Read the model definition and answer for the solid it produces. Units are mm, in the model's axes. Face numbers are marked on the shaded views. A direction names the side the tool comes from. Coordinates: 2 decimals unless noted, no trailing zeros. Order: outer loops, then holes, each group sorted by start corner. A loop starts at its lowest first (then second) coordinate and runs counter-clockwise, first axis right, second up. Notation, with made-up numbers: (-29.75, -7.75) - (-10.75, -7.75) arc R21 cw to (-10.75, 16.25) - close; hole circle Ø3 at (50.5, 19.5). An arc over 180 degrees is marked (long way). Write item = value, one per line.
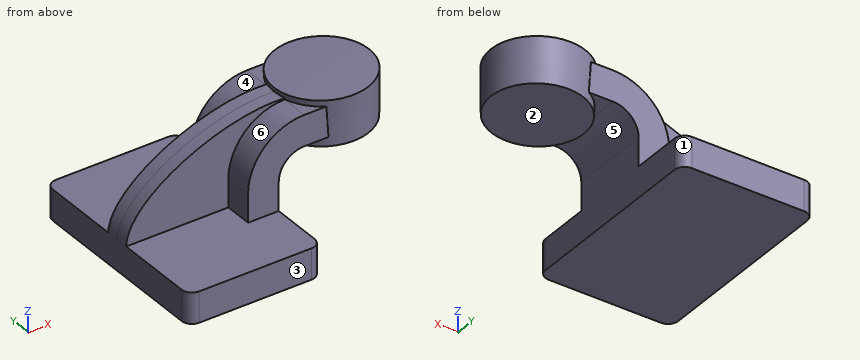
from build123d import *

# Parameters (mm, degrees)
F1_DEPTH = 63.5
F0_W     = 21.2541334692
F0_H     = 19.05
F2_DEPTH = 25.4
F3_DEPTH = 7.9375
F5_R     = 6.35


with BuildPart() as f1:
    # F0 (on Front) → F1 (new body, symmetric)
    with BuildSketch(Plane.XZ):
        Polygon((22.225, 9.525), (-41.275, 9.525), (-41.275, -9.525), (41.275, -9.525), (41.275, 9.525), align=None)
    extrude(amount=F1_DEPTH, both=True)

    # F0 (on Front) → F2 (join, symmetric)
    with BuildSketch(Plane.XZ):
        with Locations((75.0979332654, 52.4002)):
            Rectangle(F0_W, F0_H)
        with BuildLine():
            Line((22.225, 27.0002), (22.225, 9.525))
            Line((22.225, 9.525), (41.275, 9.525))
            Line((41.275, 9.525), (41.275, 27.0002))
            ThreePointArc((41.275, 27.0002), (45.9246798487, 38.2255201513), (57.15, 42.8752))
            Line((57.15, 42.8752), (64.4708665308, 42.8752))
            Line((64.4708665308, 42.8752), (64.4708665308, 61.9252))
            Line((64.4708665308, 61.9252), (57.15, 61.9252))
            ThreePointArc((57.15, 61.9252), (32.4542956671, 51.6959043329), (22.225, 27.0002))
        make_face()
    extrude(amount=F2_DEPTH, both=True)

    # F0 (on Front) → F3 (join, symmetric)
    with BuildSketch(Plane.XZ):
        with BuildLine():
            add(Edge.make_bspline(
                [(64.4708665308, 61.9252), (23.5755275935, 69.2807137966), (-40.8611632884, 37.480790168), (-41.275, 9.525)],
                knots=[0, 0, 0, 0, 118.0168176507, 118.0168176507, 118.0168176507, 118.0168176507], degree=3))
            Line((-41.275, 9.525), (22.225, 9.525))
            Line((22.225, 9.525), (22.225, 27.0002))
            ThreePointArc((22.225, 27.0002), (32.4542956671, 51.6959043329), (57.15, 61.9252))
            Line((57.15, 61.9252), (64.4708665308, 61.9252))
        make_face()
    extrude(amount=F3_DEPTH, both=True)

    # F0 (on Front) → F4 (revolve)
    with BuildSketch(Plane.XZ):
        Polygon((115.2708665308, 66.675), (85.725, 66.675), (86.3811299205, 38.1), (115.2708665308, 38.1), align=None)
    revolve(axis=Axis((86.0530649602, 0, 52.3875), (-0.0229556263, 0, 0.9997364849)))

    # F5
    f5_edges = [f1.edges().sort_by_distance(p)[0] for p in [
        (-41.275, -63.5, 0),
        (41.275, -63.5, 0),
        (41.275, 63.5, 0),
        (-41.275, 63.5, 0),
    ]]
    fillet(f5_edges, radius=F5_R)


solid = f1.part
1) For the marked faces 4, 5 and 6, determine the directions among +Z, -Z, +X, -X, +Y, -Y from which every point of the face is accessible in a straight line to the end or side of a thin tool.
Returned:
face_4 = +Z, -X, +Y
face_5 = -Z, +Y, -Y
face_6 = +Z, -X, -Y
2) Flat-ended cylindrical pins translate along their axes: pin 1 Ø16.5 at (x, y) = (67, -2.5) entering from -Z; pin 2 Ø14 at (y, z) = (15, 21) entering from -X (3 decimals); pin 3 Ø8 at (x, y) = (-7.5, 10.5) entering from +Z. Find the tip coordinate at first contact, or state that the pin passes through.
Returned:
pin_1 = 36.83
pin_2 = 22.225
pin_3 = 48.54
3) Determine the mould class of the marked faces 1, 2 and 3 for opening direction Y: pulls with the +Y half, pulls with the -Y half, needs draft (parallel to the pull), parting line crosses it, or undercut.
Returned:
face_1 = pulls with the +Y half
face_2 = undercut
face_3 = pulls with the -Y half
4) Straight lines are drawn through the part: line 1 along Y through (x, z) = (39, 46); line 2 along Y through (x, z) = (19, 29); line 3 along X through (y, z) = (-16.5, -2) (3 decimals). For each, find the intervals that lie inside material, in ascending order. Write a range as from..to.
Returned:
line_1 = -25.4..25.4
line_2 = -7.94..7.94
line_3 = -41.275..41.275
5) The part is cut by section A-A (z = 5). Determine the outline of the cut face in (x, y) (3 decimals).
Returned:
outline = (-41.275, -57.15) arc R6.35 ccw to (-34.925, -63.5) - (34.925, -63.5) arc R6.35 ccw to (41.275, -57.15) - (41.275, 57.15) arc R6.35 ccw to (34.925, 63.5) - (-34.925, 63.5) arc R6.35 ccw to (-41.275, 57.15) - close
6) The part is cut by section B-B (y = -43.5). Determine the outline of the cut face in (x, z) (3 decimals).
Returned:
outline = (-41.275, -9.525) - (41.275, -9.525) - (41.275, 9.525) - (-41.275, 9.525) - close
